Geometry check sheet. Reference: the model listing, model coordinates, mm. Face numbers are marked on the shaded views. A direction names the side the tool comes from. Give positions to 0.01 mm unless a question says otherwise; leave off trailing zeros. Write each loop counter-clockwise with the first axis right and the second up, starting at its lowest first coordinate (ties: lowest second). Pieces come first, ordered by that corner, then holes. Notation, with made-up numbers: M -16.5,34 L 35.5,34 A21 cw 35.5,67 Z; hole C 49.5,-6 d4. An arc over 180 degrees is marked long. One line per item, written item: value. Start each with the question number.
1. Scan lines: line 1 (Z direction, x = -42, y = -134); line 2 (X direction, y = -48, z = 42.75); line 3 (X direction, y = -15.5, z = 27.5). Record each from-to range of solid material in increasing order.
2. Tool access check on the marked faces 1 and 2. Record the directions out of +Z, -Z, +X, -X, +Y, -Y that give a thin tool (end or side, any length) a straight path to the whole face; none if there is none.
3. Cross-section at C-C on y = -168.5. Record the cut outline in (x, z), then the cut area to 4 significant figures.
4. Release check for a two-part mould opening along Z. For the marked faces 3, 4, 5 and 6 record: pulls with the +Z half, pulls with the -Z half, needs draft (parallel to the pull), parting line crosses it, or undercut.
5. Cross-section at A-A on z = 35. Record the cut outline in (x, y), then the cut area to 3 significant figures.
6. Cross-section at B-B on y = -114.5. Record the cut outline in (x, z), then the cut area to 4 significant figures.
7. Gauge pin test, flat end, axial feed: pin 1 (1.8 mm diameter, centred on x = -44.48, y = -104.5, fed in from -Z). Record the tip position at first contact, or that the pin passes through.
from build123d import *

# Parameters (mm, degrees)
F0_W     = 20
F0_H     = 20
F0_W_2   = 18.5
F0_H_2   = 18.5
F1_DEPTH = 240
F2_W     = 6
F2_H     = 9
F3_DEPTH = 25
F5_DEPTH = 25


with BuildPart() as f1:
    # F0 (on Front) → F1 (new body)
    with BuildSketch(Plane.XZ):
        with Locations((-44.484539, 36.999997)):
            Rectangle(F0_W, F0_H)
        with Locations((-44.484539, 36.999997)):
            Rectangle(F0_W_2, F0_H_2, mode=Mode.SUBTRACT)
    extrude(amount=F1_DEPTH)

    # F2 (on face) → F3 (cut)
    with BuildSketch(Plane.XY.offset(46.999997)):
        with Locations((-44.484539, -124.5)):
            Rectangle(F2_W, F2_H)
        with Locations((-44.484539, -115.5)):
            Rectangle(F2_W, F2_H)
        Polygon((-48.484539, -110), (-48.484539, -120), (-47.484539, -120), (-47.484539, -111), (-41.484539, -111), (-41.484539, -120), (-40.484539, -120), (-40.484539, -110), (-44.484539, -110), align=None)
        Polygon((-47.484539, -120), (-48.484539, -120), (-48.484539, -130), (-44.484539, -130), (-40.484539, -130), (-40.484539, -120), (-41.484539, -120), (-41.484539, -129), (-47.484539, -129), align=None)
        with BuildLine():
            ThreePointArc((-42.984539, -104.5), (-45.545199, -103.43934), (-44.484539, -106))
            ThreePointArc((-44.484539, -106), (-43.423879, -105.56066), (-42.984539, -104.5))
        make_face()
        with BuildLine():
            ThreePointArc((-42.984539, -135.5), (-43.423879, -134.43934), (-44.484539, -134))
            ThreePointArc((-44.484539, -134), (-45.545199, -136.56066), (-42.984539, -135.5))
        make_face()
    extrude(amount=-F3_DEPTH, mode=Mode.SUBTRACT)

    # F4 (on face) → F5 (cut)
    with BuildSketch(Plane.XY.offset(46.999997)):
        with BuildLine():
            ThreePointArc((-44.484539, -226.5), (-43.070325, -225.914214), (-42.484539, -224.5))
            ThreePointArc((-42.484539, -224.5), (-45.898752, -223.085786), (-44.484539, -226.5))
        make_face()
        with BuildLine():
            ThreePointArc((-44.484539, -13.5), (-45.898752, -16.914214), (-42.484539, -15.5))
            ThreePointArc((-42.484539, -15.5), (-43.070325, -14.085786), (-44.484539, -13.5))
        make_face()
    extrude(amount=-F5_DEPTH, mode=Mode.SUBTRACT)


solid = f1.part
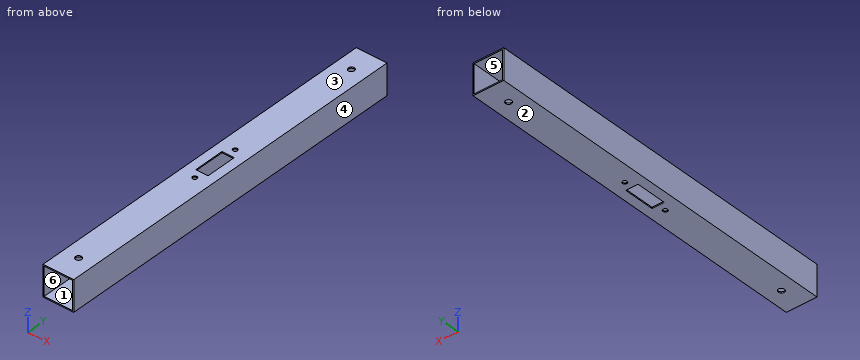
Report:
1. line 1: z = 27 to 27.75, 46.25 to 47
1. line 2: x = -54.48 to -53.73, -35.23 to -34.48
1. line 3: x = -54.48 to -46.48, -42.48 to -34.48
2. face 1: +Y, -Y
2. face 2: -Z, +X, -X, +Y, -Y
3. outline: M -54.48,27 L -34.48,27 L -34.48,47 L -54.48,47 Z; hole M -53.73,27.75 L -35.23,27.75 L -35.23,46.25 L -53.73,46.25 Z
3. area: 57.75 mm^2
4. face 3: pulls with the +Z half
4. face 4: needs draft
4. face 5: undercut
4. face 6: undercut
5. outline: M -54.48,-240 L -53.73,-240 L -53.73,0 L -54.48,0 Z; M -35.23,-240 L -34.48,-240 L -34.48,0 L -35.23,0 Z
5. area: 360 mm^2
6. outline: M -54.48,27 L -48.48,27 L -48.48,27.75 L -53.73,27.75 L -53.73,46.25 L -48.48,46.25 L -48.48,47 L -54.48,47 Z; M -40.48,27 L -34.48,27 L -34.48,47 L -40.48,47 L -40.48,46.25 L -35.23,46.25 L -35.23,27.75 L -40.48,27.75 Z
6. area: 45.75 mm^2
7. pin 1: passes through
